Source: CAD feature listing. Evaluate the final solid. Frame: model axes, mm. Face numbers are marked on the shaded views. Coordinates: 2 decimals unless noted, no trailing zeros. Write each loop counter-clockwise with the first axis right and the second up, starting at its lowest first coordinate (ties: lowest second). Pieces come first, ordered by that corner, then holes. Notation, with made-up numbers: (61, 6) - (70, 6) arc R32 cw to (70, 32) - close; hole circle Ø3 at (-21.5, -11). An arc over 180 degrees is marked (long way). One line per item, written item: value.
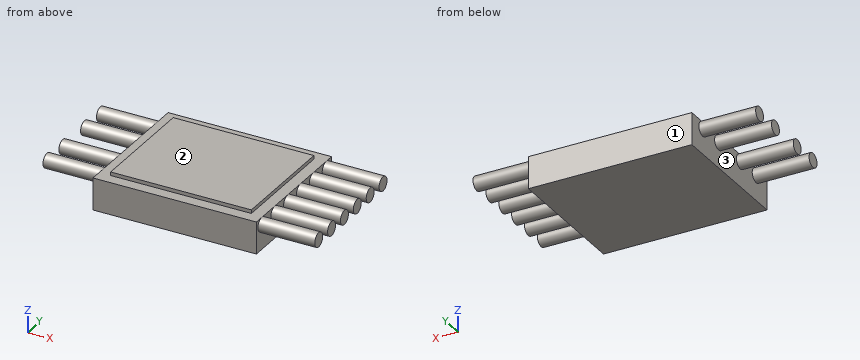
from build123d import *

# Parameters (mm, degrees)
F0_W     = 23
F0_H     = 19
F1_DEPTH = 2.5
F2_R     = 1
F3_DEPTH = 8
F4_R     = 1
F5_DEPTH = 8
F6_W     = 23
F6_H     = 19
F6_W_2   = 19.8
F6_H_2   = 15.8
F7_DEPTH = 0.5


with BuildPart() as f1:
    # F0 (on Top) → F1 (new body, symmetric)
    with BuildSketch(Plane.XY):
        Rectangle(F0_W, F0_H)
    extrude(amount=F1_DEPTH, both=True)

    # F2 (on face) → F3 (join)
    with BuildSketch(Plane.YZ.offset(11.5)):
        with Locations((-8.125, 1)):
            Circle(F2_R)
        with Locations((-4.875, 1)):
            Circle(F2_R)
        with Locations((-1.625, 1)):
            Circle(F2_R)
        with Locations((1.625, 1)):
            Circle(F2_R)
        with Locations((4.875, 1)):
            Circle(F2_R)
        with Locations((8.125, 1)):
            Circle(F2_R)
    extrude(amount=F3_DEPTH)

    # F4 (on face) → F5 (join)
    with BuildSketch(Plane(origin=(-11.5, 0, 0), x_dir=(0, -1, 0), z_dir=(-1, 0, 0))):
        with Locations((-6.75, 1)):
            Circle(F4_R)
        with Locations((-2.75, 1)):
            Circle(F4_R)
        with Locations((2.75, 1)):
            Circle(F4_R)
        with Locations((6.75, 1)):
            Circle(F4_R)
    extrude(amount=F5_DEPTH)

    # F6 (on face) → F7 (cut)
    with BuildSketch(Plane.XY.offset(2.5)):
        Rectangle(F6_W, F6_H)
        Rectangle(F6_W_2, F6_H_2, mode=Mode.SUBTRACT)
    extrude(amount=-F7_DEPTH, mode=Mode.SUBTRACT)


solid = f1.part
1) Section query C-C on y = -4.5. Output: boundary loops of the cut face in (x, z).
Values found:
outline: (-11.5, -2.5) - (11.5, -2.5) - (11.5, 0.07) - (19.5, 0.07) - (19.5, 1.93) - (11.5, 1.93) - (11.5, 2) - (9.9, 2) - (9.9, 2.5) - (-9.9, 2.5) - (-9.9, 2) - (-11.5, 2) - close
2) Draft query along Y for the marked faces 1, 2 and 3. Return one class per face: released by +Y, released by -Y, zero draft, split by the parting line, or undercut.
Values found:
face 1: released by +Y
face 2: zero draft
face 3: undercut
3) Section query D-D on z = -1.5. Output: boundary loops of the cut face in (x, y), then the cut area to 3 significant figures.
Values found:
outline: (-11.5, -9.5) - (11.5, -9.5) - (11.5, 9.5) - (-11.5, 9.5) - close
area: 437 mm2
4) Material intervals for line 1 (X direction, y = -5.5, z = 1.75); line 2 (Y direction, x = -3.5, z = 2.25); line 3 (X direction, y = -5.75, z = -0.85), sorted ascending.
Values found:
line 1: -11.5 to 19.5
line 2: -7.9 to 7.9
line 3: -11.5 to 11.5
5) Section query B-B on x = -9. Output: boundary loops of the cut face in (y, z), then the cut area to 3 significant figures.
Values found:
outline: (-9.5, -2.5) - (9.5, -2.5) - (9.5, 2) - (7.9, 2) - (7.9, 2.5) - (-7.9, 2.5) - (-7.9, 2) - (-9.5, 2) - close
area: 93.4 mm2
6) Section query A-A on x = 17.5. Output: boundary loops of the cut face in (y, z) (3 decimals), then the cut area to 3 significant figures.
Values found:
outline: circle Ø2 at (-8.125, 1); circle Ø2 at (-4.875, 1); circle Ø2 at (-1.625, 1); circle Ø2 at (1.625, 1); circle Ø2 at (4.875, 1); circle Ø2 at (8.125, 1)
area: 18.8 mm2
7) Contact query for flat-ended pins moving along their axis: P1, Ø0.6, axis at y = 3.5, z = 2.5, coming from the -X side; P2, Ø2, axis at y = 2.5, z = -1, coming from the +X side; P3, Ø5, axis at x = 14.5, y = -5.5, coming from the +Z side. Output: stop coordinate, or through.
Values found:
P1: x = -9.9
P2: x = 11.5
P3: z = 2
